from build123d import *

# Parameters (mm, degrees)
BOSS_EXTRUDE1_DEPTH = 2
SKETCH3_W           = 9
SKETCH3_H           = 50
SKETCH3_R           = 2.15
BOSS_EXTRUDE2_DEPTH = 5
FILLET1_R           = 3
BOSS_EXTRUDE3_DEPTH = 7
CUT_EXTRUDE1_REACH  = 76.971
SKETCH5_R           = 2.6
CUT_EXTRUDE2_REACH  = 79.848
SKETCH7_R           = 2.6
CUT_EXTRUDE3_DEPTH  = 7
FILLET2_R           = 1


with BuildPart() as part:
    # Sketch1 → Boss-Extrude1 (new, symmetric)
    with BuildSketch(Plane.XY):
        Polygon((0, 0), (15.5, 0), (15.5, -34.5), (24.5, -34.5), (24.5, 0), (40, 0), (40, 40), (0, 40), align=None)
    extrude(amount=BOSS_EXTRUDE1_DEPTH, both=True)

    # Sketch3 → Boss-Extrude2 (add)
    with BuildSketch(Plane.XZ.offset(34.5)):
        with Locations((20, -27)):
            Rectangle(SKETCH3_W, SKETCH3_H)
        with Locations(Location((20, -48, 0), (0, 0, 270))):
            Circle(SKETCH3_R, mode=Mode.SUBTRACT)
        with Locations(Location((20, -39, 0), (0, 0, 270))):
            Circle(SKETCH3_R, mode=Mode.SUBTRACT)
    extrude(amount=-BOSS_EXTRUDE2_DEPTH)

    # Fillet1
    fillet1_edges = [part.edges().sort_by_distance(p)[0] for p in [
        (0, 40, 0),
        (40, 40, 0),
        (40, 0, 0),
        (24.5, 0, 0),
        (15.5, 0, 0),
        (0, 0, 0),
        (20, -34.5, 2),
        (20, -29.5, -2),
    ]]
    fillet(fillet1_edges, radius=FILLET1_R)

    # Sketch4 → Boss-Extrude3 (add)
    with BuildSketch(Plane(origin=(0, 0, -2), x_dir=(-1, 0, 0), z_dir=(0, 0, -1))):
        Polygon((-20, 2.32233047), (-37.67766953, 20), (-20, 37.67766953), (-2.32233047, 20), align=None)
        Polygon((-20, 5.150757595), (-34.849242405, 20), (-20, 34.849242405), (-5.150757595, 20), align=None, mode=Mode.SUBTRACT)
    extrude(amount=BOSS_EXTRUDE3_DEPTH)

    # Cut-Extrude1: up to this face of the body (flat: up to its plane)
    cut_extrude1_end = Plane(part.part.faces().sort_by_distance((28.838834765, 28.838834765, -5.5))[0])
    # Sketch5 → Cut-Extrude1 (cut, up to the picked face)
    with BuildSketch(Plane(origin=(11.161165235, 11.161165235, 0), x_dir=(0, 0, 1), z_dir=(-0.7071067811865398, -0.7071067811865552, 0)), mode=Mode.PRIVATE) as cut_extrude1_sk1:
        with Locations(Location((-5.5, 0, 0), (0, 0, 270))):
            Circle(SKETCH5_R)
    cut_extrude1_tool1 = split(extrude(cut_extrude1_sk1.sketch, amount=-CUT_EXTRUDE1_REACH, mode=Mode.PRIVATE), bisect_by=cut_extrude1_end, keep=Keep.BOTH, mode=Mode.PRIVATE)
    add(cut_extrude1_tool1.solids().sort_by(Axis((11.161165, 11.161165, -5.5), (0.7071067811865398, 0.7071067811865552, 0)))[0], mode=Mode.SUBTRACT)

    # Cut-Extrude2: up to this face of the body (flat: up to its plane)
    cut_extrude2_end = Plane(part.part.faces().sort_by_distance((11.161165235, 28.838834765, -5.5))[0])
    # Sketch7 → Cut-Extrude2 (cut, up to the picked face)
    with BuildSketch(Plane(origin=(8.838834765, -8.838834765, 0), x_dir=(0.7071067811865399, 0.7071067811865551, 0), z_dir=(0.7071067811865551, -0.7071067811865399, 0)), mode=Mode.PRIVATE) as cut_extrude2_sk1:
        with Locations((28.284271248, -5.5)):
            Circle(SKETCH7_R)
    cut_extrude2_tool1 = split(extrude(cut_extrude2_sk1.sketch, amount=-CUT_EXTRUDE2_REACH, mode=Mode.PRIVATE), bisect_by=cut_extrude2_end, keep=Keep.BOTH, mode=Mode.PRIVATE)
    add(cut_extrude2_tool1.solids().sort_by(Axis((28.838835, 11.161165, -5.5), (-0.7071067811865551, 0.7071067811865399, 0)))[0], mode=Mode.SUBTRACT)

    # Sketch9 → Cut-Extrude3 (cut)
    with BuildSketch(Plane(origin=(0, 0, -9), x_dir=(-1, 0, 0), z_dir=(0, 0, -1))):
        Polygon((-22.828427125, 5.150757595), (-20, 2.32233047), (-17.171572875, 5.150757595), (-18.585786438, 6.564971157), (-20, 5.150757595), (-21.414213562, 6.564971157), align=None)
    extrude(amount=-CUT_EXTRUDE3_DEPTH, mode=Mode.SUBTRACT)

    # Fillet2
    fillet2_edges = [part.edges().sort_by_distance(p)[0] for p in [
        (21.414213562, 6.564971157, -5.5),
        (18.585786438, 6.564971157, -5.5),
        (17.171572875, 5.150757595, -5.5),
        (22.828427125, 5.150757595, -5.5),
        (5.150757595, 20, -5.5),
        (2.32233047, 20, -5.5),
        (20, 37.67766953, -5.5),
        (20, 34.849242405, -5.5),
        (34.849242405, 20, -5.5),
        (37.67766953, 20, -5.5),
    ]]
    fillet(fillet2_edges, radius=FILLET2_R - 0.0001)  # a hair under: the kernel refuses the full size


solid = part.part
Can you work these out from the model? Positions are in its coordinate system, mm. A direction names the side the tool comes from. Round coordinates to 2 decimals unless told otherwise and drop trailing zeros. Write each loop counter-clockwise with the first axis right and the second up, starting at its lowest first coordinate (ties: lowest second). Pieces come first, ordered by that corner, then holes. Notation, with made-up numbers: M 81.25,-16 L 109.25,-16 A19 ccw 109.25,-2 Z; hole C 17,22 d9. An arc over 180 degrees is marked long. Use a Markdown table: item, result.
Item 1: If I drill on line 1 along X through (y, z) = (-33.15, -48); line 2 along Z through (x, y) = (23, 14.5); line 3 along Y through (x, z) = (18, -4.5), over which ranges is the centre line in solid material (lowest first)? Write a range as [from, to].
Found:
| item | result |
|---|---|
| line 1 | x = [15.5, 17.85], [22.15, 24.5] |
| line 2 | z = [-2, 2] |
| line 3 | y = [-34.5, -29.46], [6, 7.13], [32.85, 35.68] |
Item 2: We'd pull the mould along Z, two halves only. Please class faces 4 (the face through (29.38, 14.53, -5.45)), 5 (the face through (29.9, 26.4, -4.7)), 6 (the face through (20, -32, -52)): released by +Z, released by -Z, zero draft, split by the parting line, or undercut.
Found:
| item | result |
|---|---|
| face 4 | zero draft |
| face 5 | undercut |
| face 6 | released by -Z |
Item 3: For pin 1 Ø5 at (x, z) = (29, -25) entering from +Y; pin 2 Ø7 at (x, z) = (18, -23.5) entering from +Y; pin 3 Ø2 at (x, z) = (7, -0.5) entering from -Y; pin 4 Ø20 at (x, y) = (12.5, 13) entering from -Z, each with a flat end and sliding along its axis, tell me the tip position at first contact or that it passes through.
Found:
| item | result |
|---|---|
| pin 1 | passes through |
| pin 2 | stops at y = -29.5 |
| pin 3 | stops at y = 0 |
| pin 4 | stops at z = -9 |
Item 4: Which directions (+Z, -Z, +X, -X, +Y, -Y) give clear straight access to the entire face, cutting with the end or side of a thin tool? Please do faces 1 (the face through (13.08, 30.76, -6.23)), 2 (the face through (8.16, 14.16, -5.45)), 3 (the face through (15.5, -30, -17)).
Found:
| item | result |
|---|---|
| face 1 | -Z, -X, +Y |
| face 2 | -Z, -X |
| face 3 | +Z, -Z, -X, -Y |
Item 5: I want a section at B-B (x = 4.5). List the corners of the cut face in (y, z) for me.
Found:
| item | result |
|---|---|
| outline | M 0,-2 L 17.82,-2 L 17.82,-9 L 22.18,-9 L 22.18,-2 L 40,-2 L 40,2 L 0,2 Z |
Item 6: I want a section at A-A (z = -39). List the corners of the cut face in (x, y) for me, and give its area (3 significant figures).
Found:
| item | result |
|---|---|
| outline | M 15.5,-34.5 L 17.85,-34.5 L 17.85,-29.5 L 15.5,-29.5 Z; M 22.15,-34.5 L 24.5,-34.5 L 24.5,-29.5 L 22.15,-29.5 Z |
| area | 23.5 mm2 |
Item 7: I want a section at C-C (y = 23). List the corners of the cut face in (x, z) for me, and give its area (3 significant figures).
Found:
| item | result |
|---|---|
| outline | M 0,-2 L 5.32,-2 L 5.32,-9 L 8.15,-9 L 8.15,-2 L 31.85,-2 L 31.85,-9 L 34.68,-9 L 34.68,-2 L 40,-2 L 40,2 L 0,2 Z |
| area | 200 mm2 |
Item 8: I want a section at D-D (z = -31). List the corners of the cut face in (x, y) for me, and give its area (3 significant figures).
Found:
| item | result |
|---|---|
| outline | M 15.5,-34.5 L 24.5,-34.5 L 24.5,-29.5 L 15.5,-29.5 Z |
| area | 45.0 mm2 |
